from build123d import *

# Parameters (mm, degrees)
SKETCH_2_W             = 16.970483697
SKETCH_2_H             = 5.016620159
CUT_EXTRUDE_1_DEPTH    = 10
CHAMFER_1_SIZE         = 1
SKETCH_3_R             = 4
EXTRUDE_1_DEPTH        = 26
FILLET_1_R             = 1
FILLET_2_R             = 0.5
CHAMFER_2_SIZE         = 0.5
HOLE_WIZARD_M3_1_D     = 2.5
HOLE_WIZARD_M3_1_DEPTH = 7.5
HOLE_WIZARD_M3_1_TIP   = 0.751075774
EXTRUDE_2_DEPTH        = 3


with BuildPart() as part:
    # 草图1 → 旋转1 (revolve)
    with BuildSketch(Plane.XY, mode=Mode.PRIVATE) as revolve_1_sk:
        Polygon((0, 0), (0, 59.7), (3, 59.7), (3, 45), (10, 45), (10, 40), (20, 40), (20, 0), align=None)
    revolve(revolve_1_sk.sketch.rotate(Axis((0, 0, 0), (0, 1, 0)), 90), axis=Axis((0, 0, 0), (0, 1, 0)))

    # 草图2 → 切除-拉伸1 (cut)
    with BuildSketch(Plane(origin=(0, 59.7, 0), x_dir=(1, 0, 0), z_dir=(0, 1, 0))):
        with Locations((-1.985722867, -4.50831008)):
            Rectangle(SKETCH_2_W, SKETCH_2_H)
    extrude(amount=-CUT_EXTRUDE_1_DEPTH, mode=Mode.SUBTRACT)

    # 倒角1
    chamfer_1_edges = [part.edges().sort_by_distance(p)[0] for p in [
        (0, 49.7, 2),
    ]]
    chamfer(chamfer_1_edges, length=CHAMFER_1_SIZE - 0.0001)  # a hair under: the kernel refuses the full size

    # 草图3 → 凸台-拉伸1 (add)
    with BuildSketch(Plane.XY):
        with Locations(Location((0, 8, 0), (0, 0, 180))):
            Circle(SKETCH_3_R)
    extrude(amount=EXTRUDE_1_DEPTH)

    # 圆角1
    fillet_1_edges = [part.edges().sort_by_distance(p)[0] for p in [
        (0, 0, 20),
    ]]
    fillet(fillet_1_edges, radius=FILLET_1_R)

    # 圆角2
    fillet_2_edges = [part.edges().sort_by_distance(p)[0] for p in [
        (4, 8, 26),
    ]]
    fillet(fillet_2_edges, radius=FILLET_2_R)

    # 倒角2
    chamfer_2_edges = [part.edges().sort_by_distance(p)[0] for p in [
        (0, 40, 20),
        (0, 45, 10),
    ]]
    chamfer(chamfer_2_edges, length=CHAMFER_2_SIZE)

    # M3 螺纹孔1
    with Locations(Plane(origin=(0, 40, 0), x_dir=(1, 0, 0), z_dir=(0, 1, 0))):
        with Locations((-12.990381057, -7.5), (12.990381057, -7.5), (0, 15)):
            Hole(HOLE_WIZARD_M3_1_D / 2, depth=HOLE_WIZARD_M3_1_DEPTH)
            with Locations((0, 0, -(HOLE_WIZARD_M3_1_DEPTH + HOLE_WIZARD_M3_1_TIP / 2))):  # 118° drill point
                Cone(0, HOLE_WIZARD_M3_1_D / 2, HOLE_WIZARD_M3_1_TIP, mode=Mode.SUBTRACT)

    # 草图8 → 凸台-拉伸2 (add)
    with BuildSketch(Plane(origin=(0, 29, 0), x_dir=(1, 0, 0), z_dir=(0, 1, 0))):
        with BuildLine():
            Line((20.025, 0), (-20.025, 0))
            ThreePointArc((-20.025, 0), (0, 20.025), (20.025, 0))
        make_face()
    extrude(amount=-EXTRUDE_2_DEPTH)


solid = part.part
Part model, mm, in its own coordinate system. A direction names the side the tool comes from. Coordinates: 2 decimals unless noted, no trailing zeros. Order: outer loops, then holes, each group sorted by start corner. A loop starts at its lowest first (then second) coordinate and runs counter-clockwise, first axis right, second up. Notation, with made-up numbers: M 51,9 L 85,9 A20 cw 85,16 Z; hole C 87,-19.5 d2. An arc over 180 degrees is marked long. One line per question, with ' | ' between items.
Q1. Slice it at C-C (z = 21). Give the cut face in (x, y).
A:
outline: C 0,8 d8
Q2. Two-plate mould, pull along X, no slides. Class faces 1 (the face through (-0.672, 36.198, -16.054)), 2 (the face through (-0.44, 27.52, -20.02)), 3 (the face through (-2.24, 45, -2.24)): +X half, -X half, draft (parallel to the pull), parting line (faces both ways), or undercut.
A:
face 1: undercut | face 2: parting line | face 3: draft
Q3. Slice it at A-A (y = 37). Give the cut face in (x, z).
A:
outline: C 0,0 d40; hole C -12.99,7.5 d2.5; hole C 0,-15 d2.5; hole C 12.99,7.5 d2.5
Q4. Drill centre lines: line 1 (X direction, y = 38, z = 7) (3 decimals); line 2 (X direction, y = 36, z = 7.5); line 3 (Y direction, x = -16.5, z = 5). Where is each one in solid material? Low to high.
A:
line 1: x = -18.735 to -14.136, -11.845 to 11.845, 14.136 to 18.735 | line 2: x = -18.54 to -14.24, -11.74 to 11.74, 14.24 to 18.54 | line 3: y = 0 to 40
Q5. 3-axis set-ups, long thin cutter, end or side, ignore diameter. For faces 4 (the face through (4, 8, 23)), 5 (the face through (-0.9, 52.25, -2.86)), 6 (the face through (0, 0, 0)): which of +Z, -Z, +X, -X, +Y, -Y reach the whole face in a straight line?
A:
face 4: +Z | face 5: +Y | face 6: +Z, -Z, +X, -X, -Y
Q6. Slice it at B-B (y = 8). Give the cut face in (x, z), and give its area (3 significant figures).
A:
outline: M -4,19.6 A20 ccw long 4,19.6 L 4,25.5 A0.5 ccw 3.5,26 L -3.5,26 A0.5 ccw -4,25.5 Z | area: 1,310 mm^2
Q7. Pin check, flat tips, straight feed: P1, Ø3, axis at y = 14.5, z = 1, coming from the +X side; P2, Ø2, axis at x = 0.5, y = 53.5, coming from the +Z side; P3, Ø12, axis at y = 23, z = 16, coming from the +X side. Stop position of each tip, or through.
A:
P1: stops at x = 20 | P2: stops at z = 2 | P3: stops at x = 17.32
Q8. Slice it at D-D (y = 53). Give the cut face in (x, z), and give its area (3 significant figures).
A:
outline: M -2.24,2 A3 ccw long 2.24,2 Z | area: 25.2 mm^2
